Read the model definition and answer for the solid it produces. Units are mm, in the model's axes. Face numbers are marked on the shaded views. A direction names the side the tool comes from. Round coordinates to 2 decimals unless told otherwise and drop trailing zeros. Write each loop counter-clockwise with the first axis right and the second up, starting at its lowest first coordinate (ties: lowest second). Pieces come first, ordered by that corner, then holes. Notation, with made-up numbers: M -12,62 L 18,62 A10 ccw 18,73 Z; hole C 70,67 d2. An arc over 180 degrees is marked long. Use one line per item in the form item = value. Start each with the question number.
```python
from build123d import *

# Parameters (mm, degrees)
BASPROSKE_W         = 3
BASPROSKE_H         = 14
TOOTHCUT_DEPTH      = 21.024984395
TEETHCUTS_COUNT     = 26
TEETHCUTS_ANGLE     = 346.153846154
BORSKE_R            = 4
BORE_DEPTH          = 50.0000508
EXTRUDE_START       = -3
SKETCH_1_R          = 4
EXTRUDE_1_DEPTH     = 3
SKETCH_2_R          = 5
CUT_EXTRUDE_1_DEPTH = 3


with BuildPart() as part:
    # BasProSke → Base-Revolve (revolve)
    with BuildSketch(Plane(origin=(0, 0, 0), x_dir=(1, 0, 0), z_dir=(0, 1, 0)), mode=Mode.PRIVATE) as base_revolve_sk:
        with Locations((1.5, 7)):
            Rectangle(BASPROSKE_W, BASPROSKE_H)
    revolve(base_revolve_sk.sketch.rotate(Axis((-10, 0, 0), (1, 0, 0)), 180), axis=Axis((-10, 0, 0), (1, 0, 0)))

    # TooCutSke → ToothCut (cut, through all)
    with BuildSketch(Plane(origin=(0, 0, 0), x_dir=(0, 0, -1), z_dir=(1, 0, 0))):
        with BuildLine():
            ThreePointArc((0.476965065, 11.739314517), (0, 11.749), (-0.476965065, 11.739314517))
            ThreePointArc((-0.476965065, 11.739314517), (-0.82065865, 12.901686978), (-1.424117301, 13.952911348))
            ThreePointArc((-1.424117301, 13.952911348), (0, 14.0254), (1.424117301, 13.952911348))
            ThreePointArc((1.424117301, 13.952911348), (0.82065865, 12.901686978), (0.476965065, 11.739314517))
        make_face()
    toothcut = extrude(amount=TOOTHCUT_DEPTH, mode=Mode.SUBTRACT)

    # TeethCuts: ToothCut ×26 about axis
    teethcuts_axis = Axis((-10, 0, 0), (1, 0, 0))
    for i in range(1, TEETHCUTS_COUNT):
        add(toothcut.rotate(teethcuts_axis, i * TEETHCUTS_ANGLE / (TEETHCUTS_COUNT - 1)), mode=Mode.SUBTRACT)

    # BorSke → Bore (cut, symmetric)
    with BuildSketch(Plane(origin=(0, 0, 0), x_dir=(0, 0, -1), z_dir=(1, 0, 0))):
        with Locations(Location((0, 0, 0), (0, 0, 180))):
            Circle(BORSKE_R)
    extrude(amount=BORE_DEPTH, both=True, mode=Mode.SUBTRACT)

    # ｽｹｯﾁ1 → ﾎﾞｽ - 押し出し1 (add)
    with BuildSketch(Plane.ZY.offset(EXTRUDE_START)):
        Circle(SKETCH_1_R)
    extrude(amount=EXTRUDE_1_DEPTH)

    # ｽｹｯﾁ2 → ｶｯﾄ - 押し出し1 (cut)
    with BuildSketch(Plane.ZY):
        Circle(SKETCH_2_R)
    extrude(amount=-CUT_EXTRUDE_1_DEPTH, mode=Mode.SUBTRACT)


solid = part.part
```
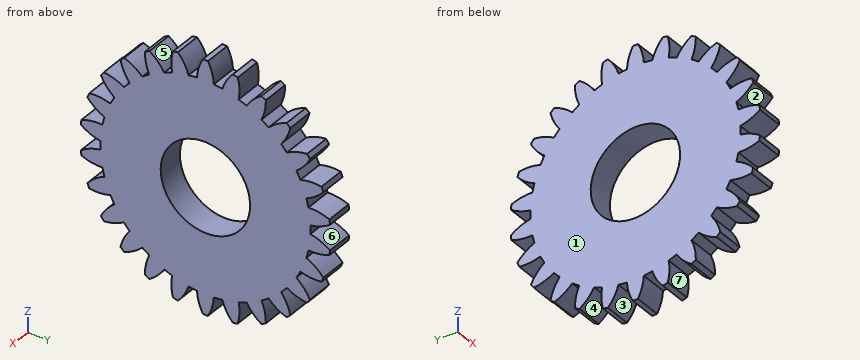
Q1. For a pull along Y with two mould halves and no side action, classify the marked faces 1, 2 and 3 as +Y half, -Y half, draft (parallel to the pull), parting line (faces both ways), or undercut.
Q2. Each of these flat-tipped pins is pushed along its axis until it touches: pin 1 Ø1.5 at (x, z) = (2.5, 5.5) entering from +Y; pin 2 Ø1.5 at (x, y) = (1.5, 8) entering from -Z; pin 3 Ø1 at (x, y) = (1.5, 2) entering from -Z. Where does it stop, or does it pass through?
Q3. Straight lines are drawn through the part: line 1 (Y direction, x = 2, z = 0); line 2 (Y direction, x = 1.75, z = -1); line 3 (Z direction, x = 1.5, y = 12.25). For each, find the intervals that lie inside material, in ascending order. Write a range as [from, to].
Q4. Find section A-A on z = 0. Write down the section's boundary in (x, y).
Q5. A tool of negligible diameter and unlimited length cuts with its end or side. For the marked faces 4, 5, 6 and 7, from which of +Z, -Z, +X, -X, +Y, -Y can it reach the whole face along a straight path? Write none if from no direction.
Q6. Find section B-B on z = -6.75. Write down the section's boundary in (x, y), and give its area (3 significant figures).
Response:
q1.face_1 = draft
q1.face_2 = -Y half
q1.face_3 = undercut
q2.pin_1 = 13.17
q2.pin_2 = -10.54
q2.pin_3 = -12.92
q3.line_1 = [-11.75, -5], [5, 11.75]
q3.line_2 = [-13.28, -4.9], [4.9, 13.28]
q3.line_3 = [-5.29, -3.82], [-2.35, -0.59], [0.59, 2.35], [3.82, 5.29]
q4.outline = M 0,-11.75 L 3,-11.75 L 3,-5 L 0,-5 Z; M 0,5 L 3,5 L 3,11.75 L 0,11.75 Z
q5.face_4 = -Z, +X, -X
q5.face_5 = +Z, +X, -X
q5.face_6 = +X, -X, +Y
q5.face_7 = +X, -X
q6.outline = M 0,-11.06 L 3,-11.06 L 3,11.06 L 0,11.06 Z
q6.area = 66.4 mm²
